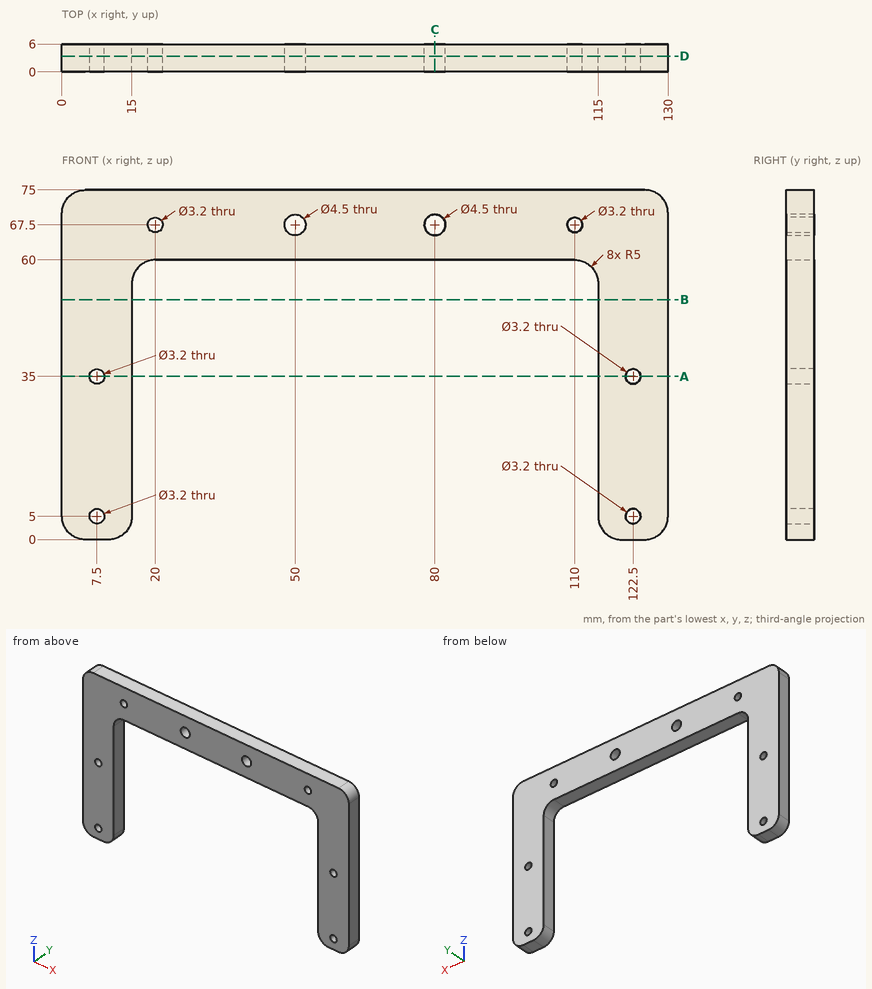
Design review of the part shown in the three views and the two pictorial views. Dimensions are in mm from the part's minimum x, y and z. Round coordinates to 2 decimals unless told otherwise and drop trailing zeros. Loops run counter-clockwise (first coordinate to the right, second up) from the corner with the lowest first, then second, coordinate; pieces in that order, holes last. Notation, with made-up numbers: (6.5, 42) -> (38.5, 42) arc R31 cw to (38.5, 72) -> close; hole circle Ø6 at (76, 69). An arc over 180 degrees is marked (long way). Return JSON: item names as keys, results as strings.
(1) Add section C-C on x = 80. Write out the cut boundary in (y, z).
Solved:
{"outline": "(0, 60) -> (6, 60) -> (6, 65.25) -> (0, 65.25) -> close; (0, 69.75) -> (6, 69.75) -> (6, 75) -> (0, 75) -> close"}
(2) Add section A-A on z = 35. Write out the cut boundary in (x, y), plus the area to 3 significant figures.
Solved:
{"outline": "(0, 0) -> (5.9, 0) -> (5.9, 6) -> (0, 6) -> close; (9.1, 0) -> (15, 0) -> (15, 6) -> (9.1, 6) -> close; (115, 0) -> (120.9, 0) -> (120.9, 6) -> (115, 6) -> close; (124.1, 0) -> (130, 0) -> (130, 6) -> (124.1, 6) -> close", "area": "142 mm2"}
(3) Add section D-D on y = 3.4. State how many separate pieces and enclosed holes the cut face has, plus the area to 3 significant figures.
Solved:
{"separate pieces": "1", "enclosed holes": "8", "area": "3,650 mm2"}
(4) For pin 1 (1.8 mm diameter, centred on x = 56.5, y = 3.5, fed in from -Z), flat-tipped, find the tip position at first contact; note if it passes through.
Solved:
{"pin 1": "z = 60"}
(5) Add section B-B on z = 51.5. Write out the cut boundary in (x, y).
Solved:
{"outline": "(0, 0) -> (15, 0) -> (15, 6) -> (0, 6) -> close; (115, 0) -> (130, 0) -> (130, 6) -> (115, 6) -> close"}
(6) For line 1 (X direction, y = 3.6, z = 5); line 2 (X direction, y = 2.35, z = 67.5); line 3 (X direction, y = 4.6, z = 15), list the stretches that pass through material, from the lowest coordinate up.
Solved:
{"line 1": "0 to 5.9, 9.1 to 15, 115 to 120.9, 124.1 to 130", "line 2": "0 to 18.4, 21.6 to 47.75, 52.25 to 77.75, 82.25 to 108.4, 111.6 to 130", "line 3": "0 to 15, 115 to 130"}
